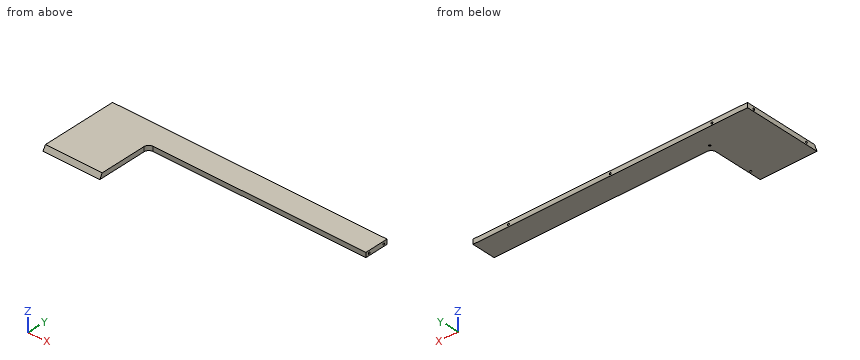
from build123d import *

# Parameters (mm, degrees)
F0_W            = 1160
F0_H            = 330
F1_DEPTH        = 20
F3_DEPTH        = 20.001
F5_DEPTH        = 580.001
F10_D           = 8
F10_DEPTH       = 30
F10_TIP         = 2.4034424761
F10_ON_F7_D     = 8
F10_ON_F7_DEPTH = 30
F10_ON_F7_TIP   = 2.4034424761
F10_ON_F8_D     = 8
F10_ON_F8_DEPTH = 30
F10_ON_F8_TIP   = 2.4034424761
F11_D           = 8
F11_DEPTH       = 10
F11_TIP         = 2.4034424761


with BuildPart() as f1:
    # F0 (on Top) → F1 (new body)
    with BuildSketch(Plane.XY):
        Rectangle(F0_W, F0_H)
    extrude(amount=F1_DEPTH)

    # F2 (on face) → F3 (cut, through all)
    with BuildSketch(Plane.XY.offset(20)):
        with BuildLine():
            Line((-340, 45), (-340, -165))
            Line((-340, -165), (580, -165))
            Line((580, -165), (580, 65))
            Line((580, 65), (-320, 65))
            ThreePointArc((-320, 65), (-334.1421356237, 59.1421356237), (-340, 45))
        make_face()
    extrude(amount=-F3_DEPTH, mode=Mode.SUBTRACT)

    # F4 (on Right) → F5 (cut, through all)
    with BuildSketch(Plane.YZ):
        Polygon((-165, 20), (-165, 0), (-153.4529946162, 20), align=None)
    extrude(amount=-F5_DEPTH, mode=Mode.SUBTRACT)

    # F10
    with Locations(Plane(origin=(-580, 0, 0), x_dir=(0, -1, 0), z_dir=(-1, 0, 0))):
        with Locations((-135, 9), (115, 9)):
            Hole(F10_D / 2, depth=F10_DEPTH)
            with Locations((0, 0, -(F10_DEPTH + F10_TIP / 2))):  # 118° drill point
                Cone(0, F10_D / 2, F10_TIP, mode=Mode.SUBTRACT)

    # F10 on F7
    with Locations(Plane(origin=(0, 165, 0), x_dir=(-1, 0, 0), z_dir=(0, 1, 0))):
        with Locations((-430, 9), (0, 9), (430, 9)):
            Hole(F10_ON_F7_D / 2, depth=F10_ON_F7_DEPTH)
            with Locations((0, 0, -(F10_ON_F7_DEPTH + F10_ON_F7_TIP / 2))):  # 118° drill point
                Cone(0, F10_ON_F7_D / 2, F10_ON_F7_TIP, mode=Mode.SUBTRACT)

    # F10 on F8
    with Locations(Plane.YZ.offset(580)):
        with Locations((80, 9), (150, 9)):
            Hole(F10_ON_F8_D / 2, depth=F10_ON_F8_DEPTH)
            with Locations((0, 0, -(F10_ON_F8_DEPTH + F10_ON_F8_TIP / 2))):  # 118° drill point
                Cone(0, F10_ON_F8_D / 2, F10_ON_F8_TIP, mode=Mode.SUBTRACT)

    # F11
    with Locations(Plane(origin=(0, 0, 0), x_dir=(1, 0, 0), z_dir=(0, 0, -1))):
        with Locations((-349, -85), (-349, 110)):
            Hole(F11_D / 2, depth=F11_DEPTH)
            with Locations((0, 0, -(F11_DEPTH + F11_TIP / 2))):  # 118° drill point
                Cone(0, F11_D / 2, F11_TIP, mode=Mode.SUBTRACT)


solid = f1.part
Part model, mm, in its own coordinate system. Coordinates: 2 decimals unless noted, no trailing zeros. Loops run counter-clockwise (first coordinate to the right, second up) from the corner with the lowest first, then second, coordinate; pieces in that order, holes last. Notation, with made-up numbers: (-8.75, 34) -> (32.25, 34) arc R24 ccw to (32.25, 63) -> close; hole circle Ø11 at (38, -34.75). An arc over 180 degrees is marked (long way). Use a Markdown table: item, result. Add a question column.
Item 1: Flat gauge pins, fed straight in: P1, Ø7, axis at x = -349, y = -110, coming from the -Z side; P2, Ø6.5, axis at x = 430, z = 9, coming from the -Y side; P3, Ø6.5, axis at y = 150, z = 9, coming from the +X side. Where does each tip first touch, or does it go through?
Item 2: Band-saw the part on A-A on x = 470. Write the cut outline in (y, z), plus the area to 3 significant figures.
Item 3: Probe probe 1 along Z at (x, y) = (556.75, 150); probe 2 along Y at (x, z) = (-349, 7); probe 3 along Y at (x, z) = (-349, 5). List the from-to ranges inside material, lowest first.
Item 4: Band-saw the part on B-B on y = 20.5. Write the cut outline in (x, z), plus the area to 3 significant figures.
Geometry says:
| question | item | result |
|---|---|---|
| 1 | P1 | z = 10.3 |
| 1 | P2 | y = 65 |
| 1 | P3 | x = 549.55 |
| 2 | outline | (65, 0) -> (165, 0) -> (165, 20) -> (65, 20) -> close |
| 2 | area | 2,000 mm² |
| 3 | probe 1 | 0 to 5, 13 to 20 |
| 3 | probe 2 | -160.96 to -114, -106 to 81, 89 to 165 |
| 3 | probe 3 | -162.11 to -114, -106 to 81, 89 to 165 |
| 4 | outline | (-580, 0) -> (-340, 0) -> (-340, 20) -> (-580, 20) -> close |
| 4 | area | 4,800 mm² |
